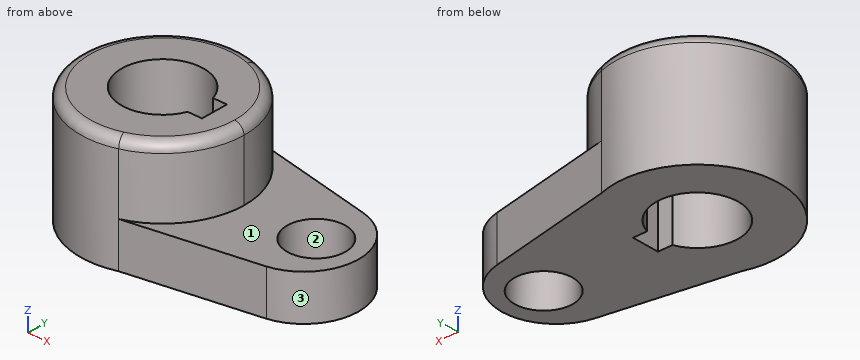
from build123d import *

# Parameters (mm, degrees)
F1_DEPTH = 40.2336
F0_R     = 10.16
F2_DEPTH = 15.7734
F3_R     = 3.302


with BuildPart() as f1:
    # F0 (on Top) → F1 (new body)
    with BuildSketch(Plane.XY):
        with BuildLine():
            ThreePointArc((-44.848745, -27.078443), (-30.766022, -16.669551), (-25.4, 0))
            ThreePointArc((-25.4, 0), (-30.766022, 16.669551), (-44.848745, 27.078443))
            ThreePointArc((-44.848745, 27.078443), (-82.55, 0), (-44.848745, -27.078443))
        make_face()
        with BuildLine():
            ThreePointArc((-40.611343, -5.054238), (-68.260442, 0.242495), (-40.4475, 4.597762))
            Line((-40.4475, 4.597762), (-35.555926, 4.597762))
            Line((-35.555926, 4.597762), (-35.555926, -5.054238))
            Line((-35.555926, -5.054238), (-40.611343, -5.054238))
        make_face(mode=Mode.SUBTRACT)
    extrude(amount=F1_DEPTH)

    # F0 (on Top) → F2 (join)
    with BuildSketch(Plane.XY):
        with BuildLine():
            ThreePointArc((-44.848745, 27.078443), (-30.766022, 16.669551), (-25.4, 0))
            ThreePointArc((-25.4, 0), (-30.766022, -16.669551), (-44.848745, -27.078443))
            Line((-44.848745, -27.078443), (0, -19.308112))
            ThreePointArc((0, -19.308112), (15.286951, -0.633478), (0, 18.041156))
            Line((0, 18.041156), (-44.848745, 27.078443))
        make_face()
        Circle(F0_R, mode=Mode.SUBTRACT)
    extrude(amount=F2_DEPTH)

    # F3
    f3_edges = [f1.edges().sort_by_distance(p)[0] for p in [
        (-63.101255, 27.078443, 40.2336),
    ]]
    fillet(f3_edges, radius=F3_R)


solid = f1.part
Can you work these out from the model? Positions are in its coordinate system, mm. Face numbers are marked on the shaded views. Give positions to 0.01 mm unless a question says otherwise; leave off trailing zeros. Loops run counter-clockwise (first coordinate to the right, second up) from the corner with the lowest first, then second, coordinate; pieces in that order, holes last. Notation, with made-up numbers: M -6.5,9 L 15.5,9 A17 cw 15.5,34 Z; hole C -17.5,63 d1. An arc over 180 degrees is marked long. One line per item, written item: value. Start each with the question number.
1) If we section it at A-A, the plane z = 11: Give the number of separate pieces and of enclosed holes in the cut face, and give its area (3 significant figures).
2) I'm going to push flat-ended pins straight in: pin 1 (1.5 mm diameter, centred on x = -38, z = 27.5, fed in from +Y); pin 2 (1.5 mm diameter, centred on y = -8.5, z = 8, fed in from +X); pin 3 (1.5 mm diameter, centred on x = -39, z = 27, fed in from -Y). Where does each tip first touch, or does it pass through?
3) If we section it at B-B, the plane x = 2: Write out the boundary of the cut face in (y, z).
4) If I drill on line 1 (X direction, y = -4, z = 8); line 2 (Y direction, x = -64.5, z = 36.5); line 3 (X direction, y = 7.5, z = 2), over which ranges is the centre line in solid material (lowest first)? Write a range as [from, to].
5) Thinking about a two-plate mould opening in Y: for the marked faces 1, 2 and 3, which applies, +Y half, -Y half, draft (parallel to the pull), parting line (faces both ways), or undercut?
Completed:
1. separate pieces: 1
1. enclosed holes: 2
1. area: 3,270 mm^2
2. pin 1: stops at y = 24.18
2. pin 2: stops at x = 13.91
2. pin 3: stops at y = -24.78
3. outline: M -18.79,0 L -9.96,0 L -9.96,15.77 L -18.79,15.77 Z; M 9.96,0 L 17.52,0 L 17.52,15.77 L 9.96,15.77 Z
4. line 1: x = [-82.27, -67.69], [-35.56, -9.34], [9.34, 14.99]
4. line 2: y = [-26.57, -9.66], [9.66, 26.57]
4. line 3: x = [-81.55, -66.14], [-41.81, -6.85], [6.85, 13.46]
5. face 1: draft
5. face 2: undercut
5. face 3: parting line
